Part model, mm, in its own coordinate system. A direction names the side the tool comes from. Round coordinates to 2 decimals unless told otherwise and drop trailing zeros. Write each loop counter-clockwise with the first axis right and the second up, starting at its lowest first coordinate (ties: lowest second). Pieces come first, ordered by that corner, then holes.
1) Saw through at B-B on y = -2.5. Write the cut outline in (x, z).
2) Which spindle directions (+Z, -Z, +X, -X, +Y, -Y) get a long thin tool onto all of the face, cutting with end or side? Do faces 5 (the flat face through (-1, -49.25, 3)), 6 (the flat face through (-25, 33, 2.5)), 7 (the flat face through (-1, 12, 0)), 8 (the cylindrical face through (22.973, -14.694, 5.768)), 9 (the flat face through (-39.65, -41.86, 3.45)). Say none if no direction does.
3) Saw through at A-A on x = 25. Write the cut outline in (y, z).
4) Saw through at C-C on y = -43. Write the cut outline in (x, z), and give its area (3 significant figures).
5) Pull direction X, two halves, no side cores. Call faces 1 (the flat face through (1, 49.25, 3)), 2 (the flat face through (39.51, -41.645, 3.451)), 3 (the cylindrical face through (-27.027, -14.694, 1.232)), 4 (the flat face through (-25, -17, 2.5)): +X half, -X half, draft (parallel to the pull), parting line (faces both ways), or undercut.
6) Drill centre lines: L1, parallel to Y at x = -25, z = 0.6; L2, parallel to X at y = -17, z = 6; L3, parallel to X at y = 31.5, z = 6.75. Where is each one in solid material? Low to high.
7) Flat gauge pins, fed straight in: pin 1 (4.5 mm diameter, centred on x = -25, y = -16.55, fed in from +Z); pin 2 (1 mm diameter, centred on y = -11, z = 4.5, fed in from +X); pin 3 (4.5 mm diameter, centred on x = 25, y = 33, fed in from -Z). Where does each tip first touch, or does it go through?
```python
from build123d import *

# Parameters (mm, degrees)
BOSS_EXTRUDE1_DEPTH = 7
CUT_EXTRUDE1_DEPTH  = 10
SKETCH3_R           = 2.75
CUT_EXTRUDE2_DEPTH  = 2.5


with BuildPart() as part:
    # Sketch1 → Boss-Extrude1 (new body)
    with BuildSketch(Plane.XY):
        Polygon((-84.25, 41.208366892), (-44.473549128, -49.25), (44.473549128, -49.25), (84.25, 41.208366892), (84.25, 49.25), (-84.25, 49.25), align=None)
    extrude(amount=BOSS_EXTRUDE1_DEPTH)

    # Sketch2 → Cut-Extrude1 (cut)
    with BuildSketch(Plane(origin=(0, 0, 0), x_dir=(-1, 0, 0), z_dir=(0, 0, -1))):
        Polygon((44.473549128, -49.25), (34.683249526, -34.25), (64.804143572, 34.25), (84.25, 41.208366892), align=None)
        Polygon((-64.804143572, 34.25), (-34.683249526, -34.25), (-44.473549128, -49.25), (-84.25, 41.208366892), align=None)
    extrude(amount=-CUT_EXTRUDE1_DEPTH, mode=Mode.SUBTRACT)

    # Sketch3 → Cut-Extrude2 (cut)
    with BuildSketch(Plane.XY.offset(7)):
        with Locations((25, 33.446923075)):
            Circle(SKETCH3_R)
        with Locations((-25, 33.446923075)):
            Circle(SKETCH3_R)
        with Locations((-25, -16.553076925)):
            Circle(SKETCH3_R)
        with Locations((25, -16.553076925)):
            Circle(SKETCH3_R)
    cut_extrude2 = extrude(amount=-CUT_EXTRUDE2_DEPTH, mode=Mode.SUBTRACT)

    # Mirror1: Cut-Extrude2 across plane
    add(cut_extrude2.mirror(Plane(origin=(0, 0, 3.5), x_dir=(1, 0, 0), z_dir=(0, 0, -1))), mode=Mode.SUBTRACT)


solid = part.part
```
Completed:
1. outline: (-48.64, 0) - (48.64, 0) - (48.64, 7) - (-48.64, 7) - close
2. face 5: +Z, -Z, +X, -X, -Y
2. face 6: -Z
2. face 7: -Z, +X, -X, +Y, -Y
2. face 8: +Z
2. face 9: +Z, -Z, -X
3. outline: (-49.25, 0) - (-19.3, 0) - (-19.3, 2.5) - (-13.8, 2.5) - (-13.8, 0) - (30.7, 0) - (30.7, 2.5) - (36.2, 2.5) - (36.2, 0) - (49.25, 0) - (49.25, 7) - (36.2, 7) - (36.2, 4.5) - (30.7, 4.5) - (30.7, 7) - (-13.8, 7) - (-13.8, 4.5) - (-19.3, 4.5) - (-19.3, 7) - (-49.25, 7) - close
4. outline: (-40.39, 0) - (40.39, 0) - (40.39, 7) - (-40.39, 7) - close
4. area: 566 mm2
5. face 1: draft
5. face 2: +X half
5. face 3: undercut
5. face 4: undercut
6. L1: y = -49.25 to -19.3, -13.8 to 30.7, 36.2 to 49.25
6. L2: x = -42.27 to -27.71, -22.29 to 22.29, 27.71 to 42.27
6. L3: x = -63.59 to -26.94, -23.06 to 23.06, 26.94 to 63.59
7. pin 1: stops at z = 4.5
7. pin 2: stops at x = 45.13
7. pin 3: stops at z = 2.5
